Check sheet for the modelled part. Datum: model origin and axes. Units: mm. Face numbers are marked on the shaded views. A direction names the side the tool comes from. Round coordinates to 2 decimals unless told otherwise and drop trailing zeros. Write each loop counter-clockwise with the first axis right and the second up, starting at its lowest first coordinate (ties: lowest second). Pieces come first, ordered by that corner, then holes. Notation, with made-up numbers: (48.25, 25.5) -> (76.25, 25.5) arc R33 cw to (76.25, 60.5) -> close; hole circle Ø7 at (-4.5, 3). An arc over 180 degrees is marked (long way). Write item = value, one per line.
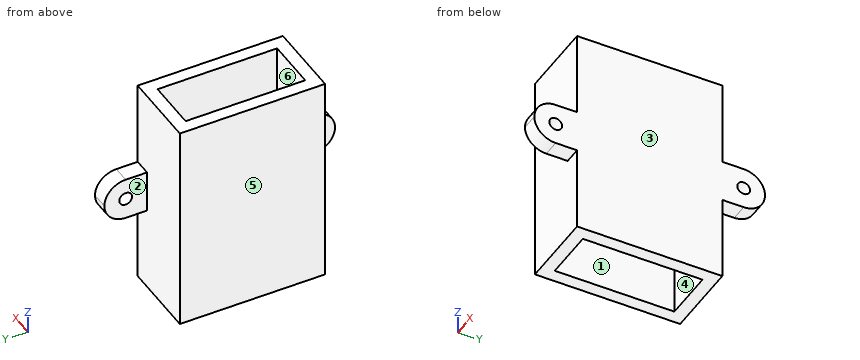
from build123d import *

# Parameters (mm, degrees)
F0_W     = 12
F0_H     = 28
F1_DEPTH = 50
F2_W     = 10
F2_H     = 10.004631
F2_R     = 1.5
F3_DEPTH = 4
F4_R     = 5
F5_R     = 5


with BuildPart() as f1:
    # F0 (on Top) → F1 (new body)
    with BuildSketch(Plane.XY):
        Polygon((-9, -17), (9, -17), (9, -5), (9, 5), (9, 17), (-9, 17), (-9, 5), (-9, -5), align=None)
        Rectangle(F0_W, F0_H, mode=Mode.SUBTRACT)
    extrude(amount=F1_DEPTH)

    # F2 (on face) → F3 (join)
    with BuildSketch(Plane.YZ.offset(9)):
        with Locations((-22, 24.997684)):
            Rectangle(F2_W, F2_H)
        with Locations((-22, 24.998842)):
            Circle(F2_R, mode=Mode.SUBTRACT)
        with Locations((22, 24.997684)):
            Rectangle(F2_W, F2_H)
        with Locations((22, 24.997685)):
            Circle(F2_R, mode=Mode.SUBTRACT)
    extrude(amount=-F3_DEPTH)

    # F4
    f4_edges = [f1.edges().sort_by_distance(p)[0] for p in [
        (7, 27, 19.995369),
        (7, 27, 30),
    ]]
    fillet(f4_edges, radius=F4_R)

    # F5
    f5_edges = [f1.edges().sort_by_distance(p)[0] for p in [
        (7, -27, 19.995369),
        (7, -27, 30),
    ]]
    fillet(f5_edges, radius=F5_R)


solid = f1.part
(1) Sectioned sample at A-A on x = 1.5. Enter the section's corners in (y, z).
Worked answers:
outline = (-17, 0) -> (-14, 0) -> (-14, 50) -> (-17, 50) -> close; (14, 0) -> (17, 0) -> (17, 50) -> (14, 50) -> close
(2) Sectioned sample at C-C on y = 18.5. Enter the section's corners in (x, z), then the cut area to 3 significant figures.
Worked answers:
outline = (5, 20) -> (9, 20) -> (9, 30) -> (5, 30) -> close
area = 40.0 mm²
(3) Sectioned sample at B-B on z = 8.5. Enter the section's corners in (x, y), then the cut area to 3 significant figures.
Worked answers:
outline = (-9, -17) -> (9, -17) -> (9, 17) -> (-9, 17) -> close; hole (-6, -14) -> (6, -14) -> (6, 14) -> (-6, 14) -> close
area = 276 mm²
(4) Go/stop test with flat-tipped pins: P1, Ø1.2, axis at x = 6.5, y = 19.5, coming from the -Z side; P2, Ø3, axis at y = 20.5, z = 25.5, coming from the -X side; P3, Ø6, axis at x = -2, z = 26.5, coming from the -Y side. Record where each tip stops, or that it passes through.
Worked answers:
P1 = 20
P2 = 5
P3 = -17
(5) Material ranges on L1, parallel to Y at x = -2.5, z = 15; L2, parallel to Z at x = 7.05, y = -22; L3, parallel to X at y = -13, z = 12, recorded low to high. Write a range as [from, to].
Worked answers:
L1 = [-17, -14], [14, 17]
L2 = [20, 23.5], [26.5, 30]
L3 = [-9, -6], [6, 9]
(6) Access from +Z, -Z, +X, -X, +Y, -Y to the whole of each face (thin tool, end or side, straight path). Record for the marked faces 1, 2 and 3.
Worked answers:
face_1 = +Z, -Z
face_2 = +Z, -Z, -X, +Y
face_3 = +Z, -Z, +X, +Y, -Y
(7) Release check for a two-part mould opening along Y. For the marked faces 4, 5 and 6 record: pulls with the +Y half, pulls with the -Y half, needs draft (parallel to the pull), parting line crosses it, or undercut.
Worked answers:
face_4 = undercut
face_5 = needs draft
face_6 = undercut
